Read the model definition and answer for the solid it produces. Units are mm, in the model's axes. A direction names the side the tool comes from. Round coordinates to 2 decimals unless told otherwise and drop trailing zeros. Loops run counter-clockwise (first coordinate to the right, second up) from the corner with the lowest first, then second, coordinate; pieces in that order, holes last. Notation, with made-up numbers: M 6.25,52.5 L 59.25,52.5 A24 cw 59.25,88.5 Z; hole C 49,-22.75 d4. An arc over 180 degrees is marked long. Write each question's results on one line, items separated by ' | '.
from build123d import *

# Parameters (mm, degrees)
BOSS_EXTRUDE1_DEPTH = 10
SKETCH2_OUTSIDE_W   = 18.56
SKETCH2_OUTSIDE_H   = 17.28
SKETCH2_OUTSIDE_R   = 4.36
CUT_EXTRUDE4_DEPTH  = 32.921929766
SKETCH3_R           = 2.384318612
CUT_EXTRUDE7_DEPTH  = 0.5
CUT_EXTRUDE8_DEPTH  = 2.5
SKETCH5_OUTSIDE_W   = 17.208
SKETCH5_OUTSIDE_H   = 17.208
SKETCH5_OUTSIDE_R   = 2.5
CUT_EXTRUDE9_DEPTH  = 25


with BuildPart() as part:
    # Sketch1 → Boss-Extrude1 (new body)
    with BuildSketch(Plane(origin=(0, 0, 0), x_dir=(0, 0, -1), z_dir=(1, 0, 0))):
        Polygon((11.5, -2.5), (-12.5, -2.5), (-12.5, -3.36), (-13.5, -4.36), (-17, -4.36), (-17.5, -3.86), (-17.5, 3.86), (-17, 4.36), (-13.5, 4.36), (-12.5, 3.36), (-12.5, 2.5), (11.5, 2.5), (12.5, 1.5), (12.5, -1.5), align=None)
    extrude(amount=BOSS_EXTRUDE1_DEPTH)

    # Sketch2 outside → Cut-Extrude4 (cut, through all)
    with BuildSketch(Plane.XY.offset(17.5)):
        with Locations((5, 0)):
            Rectangle(SKETCH2_OUTSIDE_W, SKETCH2_OUTSIDE_H)
        with Locations(Location((4.36, 0, 0), (0, 0, 339.876996719))):
            Circle(SKETCH2_OUTSIDE_R, mode=Mode.SUBTRACT)
    extrude(amount=-CUT_EXTRUDE4_DEPTH, mode=Mode.SUBTRACT)

    # Sketch3 → Cut-Extrude7 (cut)
    with BuildSketch(Plane.XY.offset(17.5)):
        with Locations((4.36, 0)):
            Circle(SKETCH3_R)
    extrude(amount=-CUT_EXTRUDE7_DEPTH, mode=Mode.SUBTRACT)

    # Sketch4 → Cut-Extrude8 (cut)
    with BuildSketch(Plane.XY.offset(17)):
        Polygon((4.36, 2.384318612), (2.295119511, 1.192159306), (2.295119511, -1.192159306), (4.36, -2.384318612), (6.424880489, -1.192159306), (6.424880489, 1.192159306), align=None)
    extrude(amount=-CUT_EXTRUDE8_DEPTH, mode=Mode.SUBTRACT)

    # Sketch5 outside → Cut-Extrude9 (cut)
    with BuildSketch(Plane(origin=(0, 0, -12.5), x_dir=(-1, 0, 0), z_dir=(0, 0, -1))):
        with Locations((-4.36, 0)):
            Rectangle(SKETCH5_OUTSIDE_W, SKETCH5_OUTSIDE_H)
        with Locations((-4.36, 0)):
            Circle(SKETCH5_OUTSIDE_R, mode=Mode.SUBTRACT)
    extrude(amount=-CUT_EXTRUDE9_DEPTH, mode=Mode.SUBTRACT)


solid = part.part
Item 1: Straight lines are drawn through the part: line 1 (X direction, y = 0, z = 17.35); line 2 (Y direction, x = 2.5, z = 15); line 3 (Z direction, x = 4.25, y = 0). For each, find the intervals that lie inside material, in ascending order.
Outcome:
line 1: x = 0 to 1.98, 6.74 to 8.72 | line 2: y = -3.94 to -1.31, 1.31 to 3.94 | line 3: z = -12.5 to 14.5
Item 2: The part is cut by section C-C (z = 1.5). Determine the outline of the cut face in (x, y).
Outcome:
outline: C 4.36,0 d5
Item 3: For faces 4 (the face through (4, 0, 14.5)), 5 (the face through (4, 0, -12.5)), 6 (the face through (6.344, -1.521, -0.175)), determine the directions among +Z, -Z, +X, -X, +Y, -Y from which every point of the face is accessible in a straight line to the end or side of a thin tool.
Outcome:
face 4: +Z | face 5: -Z, +X, -X, +Y, -Y | face 6: -Z
Item 4: The part is cut by section A-A (y = 0). Determine the outline of the cut face in (x, z).
Outcome:
outline: M 0,12.5 L 1.86,12.5 L 1.86,-12.5 L 6.86,-12.5 L 6.86,12.5 L 8.72,12.5 L 8.72,17.5 L 6.74,17.5 L 6.74,17 L 6.42,17 L 6.42,14.5 L 2.3,14.5 L 2.3,17 L 1.98,17 L 1.98,17.5 L 0,17.5 Z
Item 5: The mould has two halves that part along Y. Classify faces 1 (the face through (2.008, -3.671, 15.035)), 2 (the face through (4.32, -3.74, 12.88)), 3 (the face through (3.342, 1.797, 15.768)): pulls with the +Y half, pulls with the -Y half, needs draft (parallel to the pull), parting line crosses it, or undercut.
Outcome:
face 1: parting line crosses it | face 2: pulls with the -Y half | face 3: undercut
Item 6: Flat-ended cylindrical pins translate along their axes: pin 1 (5 mm diameter, centred on x = 4, z = 11.5, fed in from -Y); pin 2 (0.7 mm diameter, centred on y = 0.5, z = 15, fed in from -X); pin 3 (0.6 mm diameter, centred on x = 3.5, y = 1.5, fed in from +Z); pin 4 (3 mm diameter, centred on x = 5.5, z = 8, fed in from +Y). Find the tip coordinate at first contact, or state that the pin passes through.
Outcome:
pin 1: stops at y = -4.36 | pin 2: stops at x = 0 | pin 3: stops at z = 14.5 | pin 4: stops at y = 2.5
Item 7: The part is cut by section D-D (x = 6). Determine the outline of the cut face in (y, z).
Outcome:
outline: M -4.04,13.18 L -3.36,12.5 L -1.89,12.5 L -1.89,-12.11 L -1.5,-12.5 L 1.5,-12.5 L 1.89,-12.11 L 1.89,12.5 L 3.36,12.5 L 4.04,13.18 L 4.04,17.32 L 3.86,17.5 L 1.73,17.5 L 1.73,17 L 1.44,17 L 1.44,14.5 L -1.44,14.5 L -1.44,17 L -1.73,17 L -1.73,17.5 L -3.86,17.5 L -4.04,17.32 Z
Item 8: The part is cut by section B-B (x = 3.75). Determine the outline of the cut face in (y, z).
Outcome:
outline: M -4.32,13.46 L -3.36,12.5 L -2.42,12.5 L -2.42,-11.58 L -1.5,-12.5 L 1.5,-12.5 L 2.42,-11.58 L 2.42,12.5 L 3.36,12.5 L 4.32,13.46 L 4.32,17.04 L 3.86,17.5 L 2.3,17.5 L 2.3,17 L 2.03,17 L 2.03,14.5 L -2.03,14.5 L -2.03,17 L -2.3,17 L -2.3,17.5 L -3.86,17.5 L -4.32,17.04 Z
